Input: part model. Units: mm. Frame: model coordinates. Give positions to 0.01 mm unless a question says otherwise; leave off trailing zeros. Loops run counter-clockwise (first coordinate to the right, second up) from the corner with the lowest first, then second, coordinate; pieces in that order, holes last. Notation, with made-up numbers: (58, 51.5) - (92, 51.5) arc R10 ccw to (92, 64.5) - close; hole circle Ø8 at (-22, -13.75). An arc over 180 degrees is marked (long way). Answer as a JSON object with one key per item and string values. Group by question number.
(1) Section query C-C (z = -12.5). Return loops of the section in (x, y), plus the area to 3 significant figures.
(2) Section query D-D (y = 8.75). Return loops of the section in (x, z).
(3) Material intervals for L1, parallel to Z at x = 8.25, y = 6; L2, parallel to X at y = 8, z = 5.75; L3, parallel to X at y = 1, z = -6.5, sorted ascending.
(4) Mould query, pull axis X, two halves, no side actions, for faces 1 (the flat face through (0, 5, 15)), 2 (the flat face through (15, 5, 0)), 3 (the cylindrical face through (-11.93, 5.07, 11.83)). Classes: +X half, -X half, draft (parallel to the pull), parting line (faces both ways), or undercut.
(5) Section query A-A (z = 0). Return loops of the section in (x, y).
(6) Section query B-B (x = 0). Return loops of the section in (y, z), plus the area to 3 significant figures.
```python
from build123d import *

# Parameters (mm, degrees)
SCHIZZO1_W                   = 30
SCHIZZO1_H                   = 30
ESTRUSIONE_ESTRUSIONE1_DEPTH = 10
SCHIZZO2_R                   = 1.5
TAGLIO_ESTRUSIONE1_DEPTH     = 24.452078799
SCHIZZO2_3_R                 = 1.5
TAGLIO_ESTRUSIONE2_DEPTH     = 24.452078799
RACCORDO2_R                  = 2
RACCORDO3_R                  = 2
TAGLIO_ESTRUSIONE4_OUTLINE_R = 14
TAGLIO_ESTRUSIONE4_DEPTH     = 10


# Read off the part's stored shape, not the designer's step: Taglio-Estrusione4
with BuildPart() as part:
    # Schizzo1 → Estrusione-Estrusione1 (new body)
    with BuildSketch(Plane(origin=(0, 0, 0), x_dir=(1, 0, 0), z_dir=(0, 1, 0))):
        Rectangle(SCHIZZO1_W, SCHIZZO1_H)
    extrude(amount=ESTRUSIONE_ESTRUSIONE1_DEPTH)

    # Schizzo2 → Taglio-Estrusione1 (cut, through all)
    with BuildSketch(Plane(origin=(0, 10, 0), x_dir=(1, 0, 0), z_dir=(0, 1, 0))):
        with Locations(Location((-12.93949084, 12.93949084, 0), (0, 0, 270))):
            Circle(SCHIZZO2_R)
    extrude(amount=-TAGLIO_ESTRUSIONE1_DEPTH, mode=Mode.SUBTRACT)

    # Schizzo2_3 → Taglio-Estrusione2 (cut, through all)
    with BuildSketch(Plane(origin=(0, 10, 0), x_dir=(1, 0, 0), z_dir=(0, 1, 0))):
        with Locations(Location((12.93949084, -12.93949084, 0), (0, 0, 270))):
            Circle(SCHIZZO2_3_R)
        with Locations(Location((-12.93949084, -12.93949084, 0), (0, 0, 270))):
            Circle(SCHIZZO2_3_R)
        with Locations(Location((12.93949084, 12.93949084, 0), (0, 0, 270))):
            Circle(SCHIZZO2_3_R)
    extrude(amount=-TAGLIO_ESTRUSIONE2_DEPTH, mode=Mode.SUBTRACT)

    # Raccordo2
    raccordo2_edges = [part.edges().sort_by_distance(p)[0] for p in [
        (-15, 5, -15),
    ]]
    fillet(raccordo2_edges, radius=RACCORDO2_R)

    # Raccordo3
    raccordo3_edges = [part.edges().sort_by_distance(p)[0] for p in [
        (15, 5, -15),
        (15, 5, 15),
        (-15, 5, 15),
    ]]
    fillet(raccordo3_edges, radius=RACCORDO3_R)

    # Taglio-Estrusione4 outline → Taglio-Estrusione4 (cut)
    with BuildSketch(Plane(origin=(0, 0, 0), x_dir=(1, 0, 0), z_dir=(0, 1, 0))):
        Circle(TAGLIO_ESTRUSIONE4_OUTLINE_R)
    extrude(amount=TAGLIO_ESTRUSIONE4_DEPTH, mode=Mode.SUBTRACT)


solid = part.part
```
Recorded:
{
 "1": {"outline": "(-15, 0) - (-14.37, 0) - (-14.37, 10) - (-15, 10) - close; (-11.51, 0) - (-6.3, 0) - (-6.3, 10) - (-11.51, 10) - close; (6.3, 0) - (11.51, 0) - (11.51, 10) - (6.3, 10) - close; (14.37, 0) - (15, 0) - (15, 10) - (14.37, 10) - close", "area": "117 mm^2"},
 "2": {"outline": "(-15, -13) arc R2 ccw to (-13, -15) - (13, -15) arc R2 ccw to (15, -13) - (15, 13) arc R2 ccw to (13, 15) - (-13, 15) arc R2 ccw to (-15, 13) - close; hole circle Ø3 at (-12.94, -12.94); hole circle Ø3 at (-12.94, 12.94); hole circle Ø28 at (0, 0); hole circle Ø3 at (12.94, -12.94); hole circle Ø3 at (12.94, 12.94)"},
 "3": {"L1": "z = -15 to -11.31, 11.31 to 15", "L2": "x = -15 to -12.76, 12.76 to 15", "L3": "x = -15 to -12.4, 12.4 to 15"},
 "4": {"face 1": "draft", "face 2": "+X half", "face 3": "undercut"},
 "5": {"outline": "(-15, 0) - (-14, 0) - (-14, 10) - (-15, 10) - close; (14, 0) - (15, 0) - (15, 10) - (14, 10) - close"},
 "6": {"outline": "(0, -15) - (10, -15) - (10, -14) - (0, -14) - close; (0, 14) - (10, 14) - (10, 15) - (0, 15) - close", "area": "20.0 mm^2"}
}
